Autodesk Inventor part; units mm, degrees
ref_plane "YZ Plane" through (0, 0, 0) normal (1, 0, 0) x (0, 1, 0)
ref_plane "XZ Plane" through (0, 0, 0) normal (0, 1, 0) x (-1, 0, 0)
ref_plane "XY Plane" through (0, 0, 0) normal (0, 0, 1) x (1, 0, 0)
sketch "Sketch1" plane through (0, 0, 0) normal (0, 0, 1) x (1, 0, 0)
  line L0 (-22, 22) -> (22, 22)
  line L1 (22, 22) -> (22, -22)
  line L2 (22, -22) -> (-22, -22)
  line L3 (-22, -22) -> (-22, 22)
  circle A0 centre (15.5, 15.5) radius 1.475
  circle A1 centre (-15.5, 15.5) radius 1.475
  circle A2 centre (15.5, -15.5) radius 1.475
  circle A3 centre (-15.5, -15.5) radius 1.475
  line L4 (-15.5, 15.5) -> (15.5, 15.5) construction
  line L5 (15.5, 15.5) -> (15.5, -15.5) construction
  circle A4 centre (0, 0) radius 11
  line L6 (-21, 21) -> (21, 21)
  line L7 (21, 21) -> (21, -21)
  line L8 (21, -21) -> (-21, -21)
  line L9 (-21, -21) -> (-21, 21)
  line L10 (21, 21) -> (22, 21)
  line L11 (-21, 21) -> (-22, 21)
  point P0 (0, 22)
  point P1 (22, 0)
  point P2 (15.5, 0)
  point P3 (0, 15.5)
  point P4 (0, 21)
  point P5 (21, 0)
  dimension "d0" = 44
  dimension "d1" = 2.95
  dimension "d4" = 31
  dimension "d7" = 31
  dimension "d10" = 22
  dimension "d11" = 42
extrude "Extrusion1" add sketch "Sketch1" along normal blind 2 contours L11 L9 L8 L7 L10 L1 L2 L3 | L6 L7 L8 L9
extrude "Extrusion2" add sketch "Sketch1" against normal blind 38 contours L11 L9 L8 L7 L10 L1 L2 L3
sketch "Sketch2" plane through (0, 0, -38) normal (0, 0, -1) x (-1, 0, 0)
  line L0 (21, -21) -> (21, 21)
  line L1 (21, -21) -> (22, -21)
  line L2 (22, 21) -> (22, -22)
  line L3 (-21, -21) -> (-21, 21)
  line L4 (-21, -21) -> (-22, -21)
  line L5 (-22, 21) -> (-22, -22)
  line L6 (21, -21) -> (-21, -21)
  line L7 (-22, -22) -> (22, -22)
  line L8 (-20, -21) -> (-20, -22)
  line L9 (20, -21) -> (20, -22)
  line L10 (-20, -21.5) -> (20, -21.5) construction
  point P0 (0, 0)
  point P1 (0, -21.5)
  dimension "d16" = 40
extrude "Extrusion3" add sketch "Sketch2" along normal blind 50 contours L9 L7 L8 L6
sketch "Sketch3" plane through (-21, -21, 0) normal (0, 1, 0) x (1, 0, 0)
  line L0 (42, 0) -> (0, 0)
  line L1 (42, 0) -> (42, 38)
  line L2 (41, 38) -> (42, 38)
  line L3 (41, 38) -> (41, 88)
  line L4 (1, 88) -> (41, 88)
  line L5 (1, 38) -> (1, 88)
  line L6 (0, 38) -> (1, 38)
  line L7 (0, 0) -> (0, 38)
  line L8 (1, 38) -> (41, 38)
  line L9 (2.5, 87) -> (39.5, 87)
  line L10 (39.5, 87) -> (39.5, 39)
  line L11 (39.5, 39) -> (2.5, 39)
  line L12 (2.5, 39) -> (2.5, 87)
  point P0 (21, 0)
  point P1 (21, 87)
  point P2 (21, 88)
  point P3 (39.5, 63)
  point P4 (41, 63)
  dimension "d19" = 48
  dimension "d20" = 37
extrude "Extrusion4" add sketch "Sketch3" along normal blind 4 contours L8 L5 L4 L3
properties part number "Motor Stand"
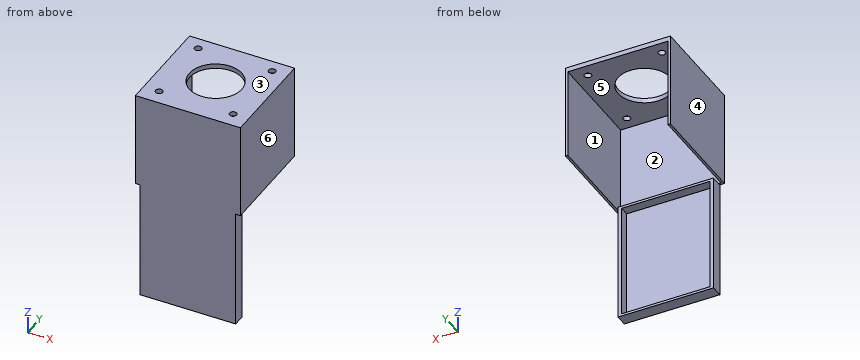
Geometry check sheet. Reference: the model listing, model coordinates, mm. Face numbers are marked on the shaded views. A direction names the side the tool comes from. Round coordinates to 2 decimals unless told otherwise and drop trailing zeros. Loops run counter-clockwise (first coordinate to the right, second up) from the corner with the lowest first, then second, coordinate; pieces in that order, holes last.
Item 1: Thickness scan on line 1 (Y direction, x = -15.5, z = 0.75) (3 decimals); line 2 (Z direction, x = 9.5, y = -20); line 3 (X direction, y = -6.5, z = -36). Record the ranges inside material, lowest first.
Item 2: Cross-section at D-D on y = 15.5. Record the boundary of the cut face in (x, z) (3 decimals).
Item 3: Access from +Z, -Z, +X, -X, +Y, -Y to the whole of each face (thin tool, end or side, straight path). Record for the marked faces 1, 2 and 3.
Item 4: Gauge pin test, flat ends, axial feed: pin 1 (5.5 mm diameter, centred on y = -20.5, z = -64.5, fed in from +X); pin 2 (21 mm diameter, centred on x = -10, y = -3.5, fed in from -Z); pin 3 (2.5 mm diameter, centred on x = -15.5, y = -15.5, fed in from +Z); pin 4 (20 mm diameter, centred on x = -7.5, z = -64.5, fed in from +Y). Record the tip position at first contact, or that the pin passes through.
Item 5: Cross-section at A-A on x = 0. Record the boundary of the cut face in (y, z).
Item 6: Cross-section at B-B on y = 0. Record the boundary of the cut face in (x, z).
Item 7: Mould release check, pull along X, two halves, no side actions. Record for the marked faces 4, 5 and 6: pulls with the +X half, pulls with the -X half, needs draft (parallel to the pull), parting line crosses it, or undercut.
Item 8: Cross-section at C-C on z = -13.5. Record the boundary of the cut face in (x, y).
Answer sheet:
1. line 1: y = -22 to -16.975, -14.025 to 14.025, 16.975 to 21
1. line 2: z = -88 to -87, -39 to -38, 0 to 2
1. line 3: x = -22 to -21, 21 to 22
2. outline: (-22, -38) - (-21, -38) - (-21, 0) - (-16.975, 0) - (-16.975, 2) - (-22, 2) - close; (-14.025, 0) - (14.025, 0) - (14.025, 2) - (-14.025, 2) - close; (16.975, 0) - (21, 0) - (21, -38) - (22, -38) - (22, 2) - (16.975, 2) - close
3. face 1: -Z, +Y
3. face 2: +Y
3. face 3: +Z, +X, -X, +Y, -Y
4. pin 1: stops at x = 20
4. pin 2: stops at z = 0
4. pin 3: passes through
4. pin 4: stops at y = -21
5. outline: (-22, -88) - (-17, -88) - (-17, -87) - (-21, -87) - (-21, -39) - (-17, -39) - (-17, -38) - (-21, -38) - (-21, 0) - (-11, 0) - (-11, 2) - (-22, 2) - close; (11, 0) - (21, 0) - (21, 2) - (11, 2) - close
6. outline: (-22, -38) - (-21, -38) - (-21, 0) - (-11, 0) - (-11, 2) - (-22, 2) - close; (11, 0) - (21, 0) - (21, -38) - (22, -38) - (22, 2) - (11, 2) - close
7. face 4: pulls with the -X half
7. face 5: undercut
7. face 6: pulls with the +X half
8. outline: (-22, -22) - (22, -22) - (22, 21) - (21, 21) - (21, -21) - (-21, -21) - (-21, 21) - (-22, 21) - close
